Autodesk Inventor part; units mm, degrees
ref_plane "YZ Plane" through (0, 0, 0) normal (1, 0, 0) x (0, 1, 0)
ref_plane "XZ Plane" through (0, 0, 0) normal (0, 1, 0) x (-1, 0, 0)
ref_plane "XY Plane" through (0, 0, 0) normal (0, 0, 1) x (1, 0, 0)
sketch "Sketch1" plane through (0, 0, 0) normal (0, 0, 1) x (1, 0, 0)
  circle A0 centre (0, 0) radius 13
  circle A1 centre (0, 0) radius 11.5
  circle A2 centre (0, 0) radius 3.15
  circle A3 centre (0, 0) radius 2
  dimension "d0" = 26
  dimension "d1" = 23
  dimension "d2" = 6.3
  dimension "d3" = 4
extrude "Extrusion1" add sketch "Sketch1" along normal blind 4 contours A0
extrude "Extrusion2" add sketch "Sketch1" along normal blind 4 contours A1 | A2 | A3
extrude "Extrusion3" add sketch "Sketch1" against normal blind 10 contours A2 | A3
extrude "Extrusion4" add sketch "Sketch1" against normal blind 25 contours A3
chamfer "Chamfer1" distance 2 angle 45 1 edges at (-13, 0, 4)
thread "Thread1"
properties part number "Manija para Bandeja"
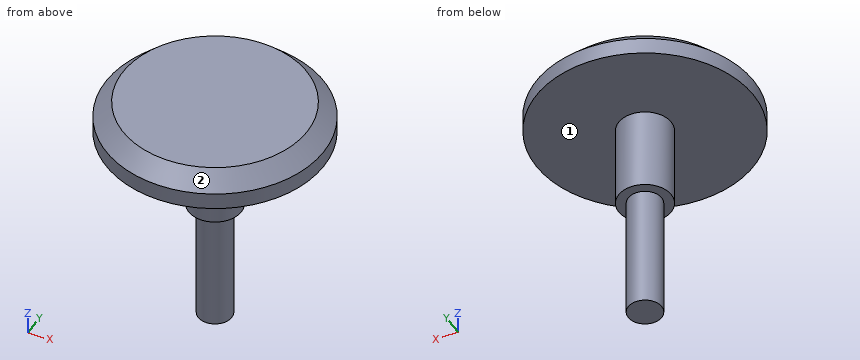
Verification items for the finished model (mm, model axes). Face numbers are marked on the shaded views. A direction names the side the tool comes from. Coordinates: 2 decimals unless noted, no trailing zeros. Order: outer loops, then holes, each group sorted by start corner. A loop starts at its lowest first (then second) coordinate and runs counter-clockwise, first axis right, second up. Notation, with made-up numbers: (-37, 43.5) -> (7, 43.5) arc R8 ccw to (7, 51.5) -> close; hole circle Ø7 at (24.25, 5.25). An arc over 180 degrees is marked (long way). Use CSV: the item, a comma, the result in double quotes. Start each with the question number.
Q1. Section check D-D, the plane z = -1.75. Record the cut outline in (x, y).
Q2. Section check C-C, the plane z = -12.25. Record the cut outline in (x, y).
Q3. Section check A-A, the plane y = 0. Record the cut outline in (x, z).
Q4. Tool access check on the marked faces 1 and 2. Record the directions out of +Z, -Z, +X, -X, +Y, -Y that give a thin tool (end or side, any length) a straight path to the whole face; none if there is none.
Q5. Thickness scan on line 1 along Z through (x, y) = (-3.25, -6.5); line 2 along Y through (x, z) = (6.25, 2); line 3 along X through (y, z) = (-7.5, 2.5). Record the ranges inside material, lowest first.
Q6. Depth check by flat-ended pin: P1, Ø1.5, axis at x = -1.5, y = 4.5, coming from the -Z side; P2, Ø4, axis at y = -3, z = -19.5, coming from the -X side; P3, Ø1.5, axis at x = -5.5, z = -0.5, coming from the -Y side. Enter the tip coordinate at first touch or a pass-through.
Returned:
1,outline,"circle Ø6.3 at (0, 0)"
2,outline,"circle Ø4 at (0, 0)"
3,outline,"(-13, 0) -> (-3.15, 0) -> (-3.15, -10) -> (-2, -10) -> (-2, -25) -> (2, -25) -> (2, -10) -> (3.15, -10) -> (3.15, 0) -> (13, 0) -> (13, 2) -> (11, 4) -> (-11, 4) -> (-13, 2) -> close"
4,face 1,"-Z"
4,face 2,"+Z"
5,line 1,"z = 0 to 4"
5,line 2,"y = -11.4 to 11.4"
5,line 3,"x = -10 to 10"
6,P1,"stops at z = 0"
6,P2,"stops at x = -1.73"
6,P3,"stops at y = -12.02"
